Here's how the part is built. I have some questions about the finished solid (model axes, mm). Face numbers are marked on the shaded views. A direction names the side the tool comes from. Coordinates: 2 decimals unless noted, no trailing zeros. Write each loop counter-clockwise with the first axis right and the second up, starting at its lowest first coordinate (ties: lowest second). Pieces come first, ordered by that corner, then holes. Notation, with made-up numbers: (27.25, 83.5) -> (68.25, 83.5) arc R12 ccw to (68.25, 96.5) -> close; hole circle Ø1 at (7.5, 35.25). An arc over 180 degrees is marked (long way). Use a Markdown table: item, result. Add a question column.
Item 1: Imagine slicing it at C-C, the plane y = 3.25. Write out the boundary of the cut face in (x, z), and give its area (3 significant figures).
Item 2: If I drill on line 1 along Z through (x, y) = (0, 2.5); line 2 along X through (y, z) = (3.1, 0.75); line 3 along Z through (x, y) = (-1.5, 2.5), over which ranges is the centre line in solid material (lowest first)? Write a range as from..to.
Item 3: Imagine slicing it at A-A, the plane x = 0. Write out the boundary of the cut face in (y, z), and give its area (3 significant figures).
Item 4: Imagine slicing it at B-B, the plane y = 0.75. Write out the boundary of the cut face in (x, z), and give its area (3 significant figures).
Item 5: Will these pins go through, and if not, where does the flat tip stop? pin 1 Ø0.5 at (x, z) = (3, -1.5) entering from +Y; pin 2 Ø3 at (x, y) = (-2.5, 4) entering from -Z; pin 3 Ø0.5 at (x, z) = (2.5, 2.5) entering from +Y.
Item 6: If we mould it in two halves opening along Z, with no side actions, what happens to the marked faces 1, 2 and 3? For each: pulls with the +Z half, pulls with the -Z half, needs draft (parallel to the pull), parting line crosses it, or undercut.
Item 7: On a 3-axis mill with a long thin cutter (end or side, diameter ignored), from which of +Z, -Z, +X, -X, +Y, -Y can I reach the whole of each face in a straight line? I mean the marked faces 4 and 5. Say none if no direction works.
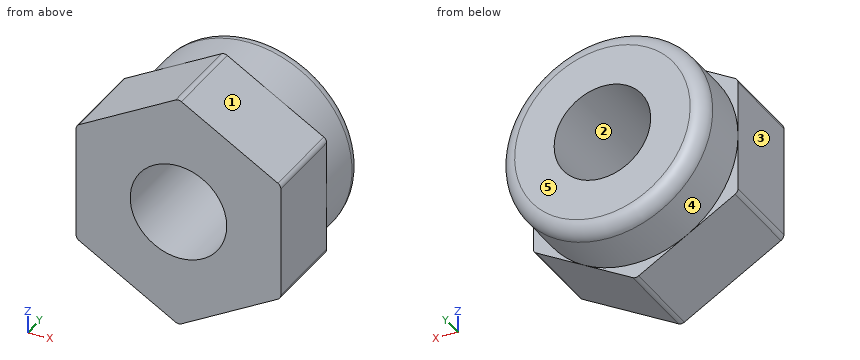
```python
from build123d import *

# Parameters (mm, degrees)
EXTRUDE_1_DEPTH    = 2.9
SKETCH_2_R         = 3.5
EXTRUDE_2_DEPTH    = 5
FILLET_1_R         = 0.5
FILLET_2_R         = 0.2
HOLE_WIZARD_M4_1_D = 3.3


with BuildPart() as part:
    # 草图1 → 凸台-拉伸1 (new body)
    with BuildSketch(Plane(origin=(0, 0, 0), x_dir=(1, 0, 0), z_dir=(0, 1, 0))):
        Polygon((0, 4.041451884), (-3.5, 2.020725942), (-3.5, -2.020725942), (0, -4.041451884), (3.5, -2.020725942), (3.5, 2.020725942), align=None)
    extrude(amount=EXTRUDE_1_DEPTH)

    # 草图2 → 凸台-拉伸2 (add)
    with BuildSketch(Plane.XZ):
        with Locations(Location((0, 0, 0), (0, 0, 270))):
            Circle(SKETCH_2_R)
    extrude(amount=-EXTRUDE_2_DEPTH)

    # 圆角1
    fillet_1_edges = [part.edges().sort_by_distance(p)[0] for p in [
        (0, 5, 3.5),
    ]]
    fillet(fillet_1_edges, radius=FILLET_1_R)

    # 圆角2
    fillet_2_edges = [part.edges().sort_by_distance(p)[0] for p in [
        (3.5, 1.45, -2.020725942),
        (3.5, 1.45, 2.020725942),
        (0, 1.45, 4.041451884),
        (-3.5, 1.45, 2.020725942),
        (-3.5, 1.45, -2.020725942),
        (0, 1.45, -4.041451884),
    ]]
    fillet(fillet_2_edges, radius=FILLET_2_R)

    # M4 螺纹孔1 (through all)
    with Locations(Plane(origin=(0, 0, 0), x_dir=(-1, 0, 0), z_dir=(0, -1, 0))):
        with Locations((0, 0)):
            Hole(HOLE_WIZARD_M4_1_D / 2)


solid = part.part
```
Ans:
| question | item | result |
|---|---|---|
| 1 | outline | circle Ø7 at (0, 0); hole circle Ø3.3 at (0, 0) |
| 1 | area | 29.9 mm^2 |
| 2 | line 1 | z = -4.01..-1.65, 1.65..4.01 |
| 2 | line 2 | x = -3.42..-1.47, 1.47..3.42 |
| 2 | line 3 | z = -3.18..-0.69, 0.69..3.18 |
| 3 | outline | (0, -4.01) -> (2.9, -4.01) -> (2.9, -3.5) -> (4.5, -3.5) arc R0.5 ccw to (5, -3) -> (5, -1.65) -> (0, -1.65) -> close; (0, 1.65) -> (5, 1.65) -> (5, 3) arc R0.5 ccw to (4.5, 3.5) -> (2.9, 3.5) -> (2.9, 4.01) -> (0, 4.01) -> close |
| 3 | area | 21.4 mm^2 |
| 4 | outline | (-3.5, -1.91) arc R0.2 ccw to (-3.4, -2.08) -> (-0.1, -3.98) arc R0.2 ccw to (0.1, -3.98) -> (3.4, -2.08) arc R0.2 ccw to (3.5, -1.91) -> (3.5, 1.91) arc R0.2 ccw to (3.4, 2.08) -> (0.1, 3.98) arc R0.2 ccw to (-0.1, 3.98) -> (-3.4, 2.08) arc R0.2 ccw to (-3.5, 1.91) -> close; hole circle Ø3.3 at (0, 0) |
| 4 | area | 33.9 mm^2 |
| 5 | pin 1 | stops at y = 4.99 |
| 5 | pin 2 | stops at z = -3.35 |
| 5 | pin 3 | stops at y = 4.91 |
| 6 | face 1 | pulls with the +Z half |
| 6 | face 2 | undercut |
| 6 | face 3 | needs draft |
| 7 | face 4 | +Y |
| 7 | face 5 | +Z, -Z, +X, -X, +Y |
